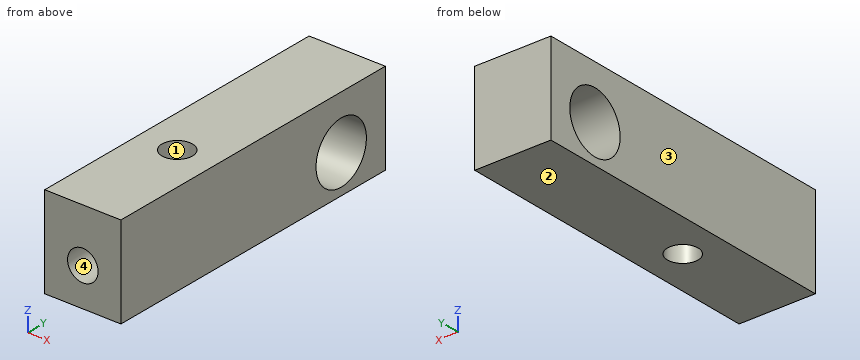
Autodesk Inventor part; units mm, degrees
ref_plane "YZ Plane" through (0, 0, 0) normal (1, 0, 0) x (0, 1, 0)
ref_plane "XZ Plane" through (0, 0, 0) normal (0, 1, 0) x (-1, 0, 0)
ref_plane "XY Plane" through (0, 0, 0) normal (0, 0, 1) x (1, 0, 0)
sketch "Esquisse1" plane through (0, 0, 0) normal (1, 0, 0) x (0, 1, 0)
  line L0 (0, 0) -> (40, 0)
  line L1 (40, 0) -> (40, -10)
  line L2 (40, -10) -> (0, -10)
  line L3 (0, -10) -> (0, 0)
  dimension "d0" = 40
  dimension "d1" = 10
extrude "Extrusion1" add sketch "Esquisse1" along normal blind 10
sketch "Esquisse2" plane through (10, 0, 0) normal (1, 0, 0) x (0, 0, -1)
  line L0 (10, 40) -> (0, 40)
  line L1 (0, 40) -> (0, 0)
  point P0 (5, 35)
  dimension "d4" = 5
  dimension "d5" = 5
hole "Perçage1" at (10, 35, -5) direction (-1, 0, 0) diameter 8 depth 10 tip angle 118
sketch "Esquisse3" plane through (0, 0, 0) normal (0, 0, 1) x (1, 0, 0)
  line L0 (0, 40) -> (0, 0)
  line L1 (10, 0) -> (10, 40)
  line L2 (0, 40) -> (10, 40)
  line L3 (10, 40) -> (10, 0)
  line L4 (10, 0) -> (0, 0)
  line L5 (0, 0) -> (0, 40)
extrude "Extrusion2" add sketch "Esquisse3" along normal blind 2
sketch "Esquisse4" plane through (0, 40, -10) normal (0, 1, 0) x (1, 0, 0)
  line L0 (0, 0) -> (0, -12)
  line L1 (0, 0) -> (10, 0)
  line L2 (0, -12) -> (10, -12)
  line L3 (10, -12) -> (10, 0)
  line L4 (10, 0) -> (0, 0)
  line L5 (0, 0) -> (0, -12)
  point P0 (0, -10)
extrude "Extrusion3" add sketch "Esquisse4" along normal blind 2
sketch "Esquisse5" plane through (10, 0, 0) normal (1, 0, 0) x (0, 0, -1)
  point P0 (0, 0)
sketch "Esquisse6" plane through (0, 0, -10) normal (0, -1, 0) x (1, 0, 0)
  line L0 (0, 0) -> (10, 0)
  line L1 (0, 0) -> (0, 12)
  point P0 (0, 10)
  point P1 (5, 5)
  dimension "d17" = 5
  dimension "d18" = 5
hole "Perçage2" at (5, 0, -5) direction (0, 1, 0) diameter 4 depth 6 tip angle 118
sketch "Esquisse7" plane through (10, 0, -10) normal (0, 0, -1) x (-1, 0, 0)
  line L0 (10, 0) -> (0, 0)
  line L1 (0, 0) -> (0, 42)
  point P0 (5, 15)
  dimension "d26" = 15
  dimension "d27" = 5
hole "Perçage3" at (5, 15, -10) direction (0, 0, 1) diameter 4 depth 12 tip angle 118
properties part number "SupportCodeuse"
Source: CAD feature listing. Evaluate the final solid. Frame: model axes, mm. Face numbers are marked on the shaded views. Coordinates: 2 decimals unless noted, no trailing zeros. Write each loop counter-clockwise with the first axis right and the second up, starting at its lowest first coordinate (ties: lowest second). Pieces come first, ordered by that corner, then holes. Notation, with made-up numbers: M 67,16 L 99,16 A13 cw 99,26 Z; hole C -10.75,62 d1. An arc over 180 degrees is marked long. Answer as a JSON object with one key per item and string values.
1. Cut plane D-D on y = 15. Output: boundary loops of the cut face in (x, z).
Evaluation:
{"outline": "M 0,-10 L 3,-10 L 3,2 L 0,2 Z; M 7,-10 L 10,-10 L 10,2 L 7,2 Z"}
2. Cut plane B-B on x = 9.25. Output: boundary loops of the cut face in (y, z), plus the area to 3 significant figures.
Evaluation:
{"outline": "M 0,-10 L 42,-10 L 42,2 L 0,2 Z; hole C 35,-5 d8", "area": "454 mm^2"}
3. Cut plane A-A on y = 35. Output: boundary loops of the cut face in (x, z).
Evaluation:
{"outline": "M 0,-10 L 10,-10 L 10,-9 L 0,-9 Z; M 0,-1 L 10,-1 L 10,2 L 0,2 Z"}
4. Draft query along X for the marked faces 1, 2, 3 and 4. Return one class per face: released by +X, released by -X, zero draft, split by the parting line, or undercut.
Evaluation:
{"face 1": "undercut", "face 2": "zero draft", "face 3": "released by -X", "face 4": "undercut"}
5. Contact query for a flat-ended pin moving along its axis: P1, Ø5, axis at y = 9, z = -0.5, coming from the -X side. Output: stop coordinate, or through.
Evaluation:
{"P1": "x = 0"}
6. Ray query, L1, parallel to Z at x = 5, y = 1.2; L2, parallel to Y at x = 2.75, z = -5; L3, parallel to Y at x = 5, z = -1.5. Return the intervals inside material, ascending.
Evaluation:
{"L1": "-10 to -7, -3 to 2", "L2": "0 to 31, 39 to 42", "L3": "0 to 13, 17 to 33.06, 36.94 to 42"}
7. Cut plane C-C on z = 0.25. Output: boundary loops of the cut face in (x, y), plus the area to 3 significant figures.
Evaluation:
{"outline": "M 0,0 L 10,0 L 10,42 L 0,42 Z; hole C 5,15 d4", "area": "407 mm^2"}
